from build123d import *

# Parameters (mm, degrees)
F1_DEPTH = 40
F3_DEPTH = 40
F6_DEPTH = 10


with BuildPart() as f1:
    # F0 (on Top) → F1 (new body)
    with BuildSketch(Plane.XY):
        with BuildLine():
            ThreePointArc((13.856406, 8), (0, -16), (-13.856406, 8))
            Line((-13.856406, 8), (-15.545047, 10.924812))
            ThreePointArc((-15.545047, 10.924812), (0, -19), (15.545047, 10.924812))
            Line((15.545047, 10.924812), (13.856406, 8))
        make_face()
    extrude(amount=F1_DEPTH)

    # F2 (on Top) → F3 (join, through all)
    with BuildSketch(Plane.XY):
        with BuildLine():
            Line((15.949585, 18.5), (13.710013, 20.739573))
            ThreePointArc((13.710013, 20.739573), (12.115595, 14.350623), (13.856406, 8))
            Line((13.856406, 8), (16.454483, 9.5))
            ThreePointArc((16.454483, 9.5), (15.130436, 13.939884), (15.949585, 18.5))
        make_face()
    extrude(amount=F3_DEPTH)

    # F4: F1 across plane


with BuildPart() as f1_1:
    add(f1.part)
    add(f1.part.mirror(Plane.YZ))

    # F5 (on face) → F6 (join)
    with BuildSketch(Plane(origin=(0, 0, 0), x_dir=(1, 0, 0), z_dir=(0, 0, -1))):
        with BuildLine():
            ThreePointArc((-18.730344, 3.189705), (0, 19), (18.730344, 3.189705))
            Line((18.730344, 3.189705), (15, 25.09475))
            ThreePointArc((15, 25.09475), (0, 27), (-15, 25.09475))
            Line((-15, 25.09475), (-18.730344, 3.189705))
        make_face()
    extrude(amount=-F6_DEPTH)


solid = f1_1.part
Part model, mm, in its own coordinate system. A direction names the side the tool comes from. Coordinates: 2 decimals unless noted, no trailing zeros. Write each loop counter-clockwise with the first axis right and the second up, starting at its lowest first coordinate (ties: lowest second). Pieces come first, ordered by that corner, then holes. Notation, with made-up numbers: M -18.5,24 L -6.5,24 A31 cw -6.5,59 Z; hole C -0.75,-20.5 d7. An arc over 180 degrees is marked long. Return JSON: item names as keys, results as strings.
1. Saw through at B-B, the plane z = 19. Write the cut outline in (x, y), then the cut area to 3 significant figures.
Determined:
{"outline": "M -16.45,9.5 A19 ccw long 16.45,9.5 A10 cw 15.95,18.5 L 13.71,20.74 A13 ccw 13.86,8 A16 cw long -13.86,8 A13 ccw -13.71,20.74 L -15.95,18.5 A10 cw Z", "area": "288 mm²"}
2. Saw through at D-D, the plane x = 0. Write the cut outline in (y, z), then the cut area to 3 significant figures.
Determined:
{"outline": "M -27,0 L -16,0 L -16,40 L -19,40 L -19,10 L -27,10 Z", "area": "200 mm²"}
3. Flat gauge pins, fed straight in: pin 1 Ø12 at (y, z) = (-8.5, 22) entering from +X; pin 2 Ø2 at (x, z) = (6.5, 35.5) entering from +Y; pin 3 Ø1.5 at (x, z) = (-15, 33) entering from -Y. Where does each tip first touch, or does it go through?
Determined:
{"pin 1": "x = 18.83", "pin 2": "y = -14.13", "pin 3": "y = -12.57"}
4. 3-axis set-ups, long thin cutter, end or side, ignore diameter. For faces 1 (the face through (0, -21, 10)), 2 (the face through (12.115, 14.444, 19.72)), 3 (the face through (-0.56, -18.99, 24.16)): which of +Z, -Z, +X, -X, +Y, -Y reach the whole face in a straight line?
Determined:
{"face 1": "+Z, -Y", "face 2": "+Z, -Z", "face 3": "+Z"}
5. Probe L1, parallel to X at y = 15, z = 30; L2, parallel to X at y = 0, z = 29.5; L3, parallel to Y at x = 13.5, z = 7. List the from-to ranges inside material, lowest first.
Determined:
{"L1": "-15.13 to -12.12, 12.12 to 15.13", "L2": "-19 to -16, 16 to 19", "L3": "-25.46 to -8.59, 8.66 to 20.34"}
6. Saw through at C-C, the plane x = 13. Write the cut outline in (y, z).
Determined:
{"outline": "M -25.57,0 L -9.33,0 L -9.33,40 L -13.86,40 L -13.86,10 L -25.57,10 Z; M 9.78,0 L 19.22,0 L 19.22,40 L 9.78,40 Z"}
7. Pull direction X, two halves, no side cores. Call faces 4 (the face through (16.89, -13.99, 4.93)), 5 (the face through (0, -16, 20)), 6 (the face through (-14.85, 19.6, 19.72)): pulls with the +X half, pulls with the -X half, needs draft (parallel to the pull), parting line crosses it, or undercut.
Determined:
{"face 4": "pulls with the +X half", "face 5": "undercut", "face 6": "pulls with the -X half"}
8. Saw through at A-A, the plane y = 0. Write the cut outline in (x, z).
Determined:
{"outline": "M -19,0 L -16,0 L -16,40 L -19,40 Z; M 16,0 L 19,0 L 19,40 L 16,40 Z"}
